Autodesk Inventor part; units mm, degrees
ref_plane "YZ Plane" through (0, 0, 0) normal (1, 0, 0) x (0, 1, 0)
ref_plane "XZ Plane" through (0, 0, 0) normal (0, 1, 0) x (-1, 0, 0)
ref_plane "XY Plane" through (0, 0, 0) normal (0, 0, 1) x (1, 0, 0)
sketch "Sketch1" plane through (0, 0, 0) normal (0, 0, 1) x (1, 0, 0)
  line L0 (0, 0) -> (63.5, 0)
  line L1 (63.5, 0) -> (63.5, 40)
  line L2 (63.5, 40) -> (0, 40)
  line L3 (0, 40) -> (0, 0)
  dimension "d2" = 40
  dimension "d3" = 63.5
extrude "Extrusion1" add sketch "Sketch1" along normal blind 6.35
sketch "Sketch2" plane through (0, 0, 6.35) normal (0, 0, 1) x (1, 0, 0)
  line L0 (0, 0) -> (0, 40)
  line L1 (0, 40) -> (63.5, 40)
  line L2 (50.8, 20) -> (12.7, 20)
  point P0 (0, 20)
  point P1 (31.75, 20)
  point P2 (31.75, 40)
  dimension "d4" = 38.1
hole "Hole1" at (12.7, 20, 6.35) at (50.8, 20, 6.35) direction (0, 0, -1) diameter 6.604 end through all
sketch "Sketch3" plane through (63.5, 0, 0) normal (1, 0, 0) x (0, 0, -1)
  line L0 (-6.35, 40) -> (-6.35, 0)
  line L1 (0, 0) -> (-6.35, 0)
  line L2 (0, 0) -> (0, 40)
  circle A0 centre (-25.4, -3.175) radius 6.35
  line L3 (0, 0) -> (-23.0739, -9.0836)
  line L4 (-30.8119, 0.1468) -> (-6.35, 40)
  dimension "d12" = 12.7
  dimension "d13" = 3.175
  dimension "d14" = 25.4
extrude "Extrusion2" add sketch "Sketch3" against normal up to surface (63.5 mm away)
sketch "Sketch4" plane through (0, 40, 0) normal (0, 1, 0) x (1, 0, 0)
  line L0 (0, -6.35) -> (63.5, -6.35)
  line L1 (63.5, 0) -> (63.5, -6.35)
  line L2 (0, 0) -> (0, -6.35)
  line L3 (6.35, -6.35) -> (57.15, -6.35)
  line L4 (57.15, -6.35) -> (57.15, -38.1)
  line L5 (57.15, -38.1) -> (6.35, -38.1)
  line L6 (6.35, -38.1) -> (6.35, -6.35)
  dimension "d17" = 31.75
  dimension "d18" = 6.35
  dimension "d19" = 6.35
extrude "Extrusion3" cut sketch "Sketch4" against normal through all
hole "Hole2" at (63.5, -3.175, 25.4) direction (-1, 0, 0) diameter 6.7564 end through all
properties part number "kinect bracket b"
Work out the finished part from the listing and answer in its coordinate system (mm). A direction names the side the tool comes from. Coordinates: 2 decimals unless noted, no trailing zeros. Order: outer loops, then holes, each group sorted by start corner. A loop starts at its lowest first (then second) coordinate and runs counter-clockwise, first axis right, second up. Notation, with made-up numbers: (39.25, 55.5) - (71.25, 55.5) arc R24 cw to (71.25, 65.5) - close; hole circle Ø7 at (25.25, -24). An arc over 180 degrees is marked (long way). Put each result on its own line as item: value. Start each with the question number.
1) For a pull along Z with two mould halves and no side action, classify faces 1 (the cylindrical face through (60.369, -7.169, 30.337)), 2 (the cylindrical face through (60.281, -3.324, 28.775)), 3 (the flat face through (32.19, -1.45, 3.68)) as released by +Z, released by -Z, zero draft, split by the parting line, or undercut.
2) Find section D-D (z = 30). Give the vertices of the cut face in (x, y).
3) For faces 4 (the cylindrical face through (48.02, 18.22, 3.13)), 5 (the flat face through (6.35, 10, 16)), determine the directions among +Z, -Z, +X, -X, +Y, -Y from which every point of the face is accessible in a straight line to the end or side of a thin tool.
4) Flat-ended cylindrical pins translate along their axes: pin 1 (12 mm diameter, centred on y = 10.5, z = 16, fed in from -X); pin 2 (4 mm diameter, centred on x = 6.5, z = 23.5, fed in from +Y); pin 3 (5 mm diameter, centred on x = 55, z = 18, fed in from -Y); pin 4 (2 mm diameter, centred on x = 31.5, y = 17.5, fed in from +Z). Find the tip coordinate at first contact, or state that the pin passes through.
5) Find section A-A (x = 12.7). Give the vertices of the cut face in (y, z).
6) Find section B-B (z = 24). Give the vertices of the cut face in (x, y).
7) Find the intervals of material crossed by line 1 (X direction, y = 20, z = 2); line 2 (X direction, y = 13, z = 12); line 3 (Z direction, x = 47, y = 19.5), in increasing order. Write a range as from..to.
8) Find section C-C (y = 21.5). Give the vertices of the cut face in (x, z).
Results list:
1. face 1: split by the parting line
1. face 2: undercut
1. face 3: released by -Z
2. outline: (0, -7.55) - (6.35, -7.55) - (6.35, 1.47) - (0, 1.47) - close; (57.15, -7.55) - (63.5, -7.55) - (63.5, 1.47) - (57.15, 1.47) - close
3. face 4: +Z, -Z
3. face 5: +Z, +Y, -Y
4. pin 1: stops at x = 0
4. pin 2: stops at y = 15.31
4. pin 3: stops at y = -7.59
4. pin 4: stops at z = 6.35
5. outline: (-2.5, 6.35) - (0, 0) - (16.7, 0) - (16.7, 6.35) - close; (23.3, 0) - (40, 0) - (40, 6.35) - (23.3, 6.35) - close
6. outline: (0, -9.37) - (6.35, -9.37) - (6.35, -6.25) - (0, -6.25) - close; (0, -0.1) - (6.35, -0.1) - (6.35, 11.24) - (0, 11.24) - close; (57.15, -9.37) - (63.5, -9.37) - (63.5, -6.25) - (57.15, -6.25) - close; (57.15, -0.1) - (63.5, -0.1) - (63.5, 11.24) - (57.15, 11.24) - close
7. line 1: x = 0..9.4, 16..47.5, 54.1..63.5
7. line 2: x = 0..6.35, 57.15..63.5
7. line 3: z = 0..6.35
8. outline: (0, 0) - (9.76, 0) - (9.76, 6.35) - (6.35, 6.35) - (6.35, 17.71) - (0, 17.71) - close; (15.64, 0) - (47.86, 0) - (47.86, 6.35) - (15.64, 6.35) - close; (53.74, 0) - (63.5, 0) - (63.5, 17.71) - (57.15, 17.71) - (57.15, 6.35) - (53.74, 6.35) - close
